from build123d import *

# Parameters (mm, degrees)
EXTRUDE1_DEPTH = 6


with BuildPart() as part:
    # Sketch1 → Extrude1 (new body)
    with BuildSketch(Plane(origin=(0, 0, 0), x_dir=(1, 0, 0), z_dir=(0, 1, 0))):
        Polygon((1.154700538, 2), (-1.154700538, 2), (-2.309401077, 0), (-1.154700538, -2), (1.154700538, -2), (2.309401077, 0), align=None)
    extrude(amount=EXTRUDE1_DEPTH)

    # Sketch3 → Cut-Revolve1 (revolve, cut)
    with BuildSketch(Plane(origin=(0, 0, 0), x_dir=(0, 0, -1), z_dir=(1, 0, 0)), mode=Mode.PRIVATE) as cut_revolve1_sk:
        Polygon((1.5, 6), (1, 5.5), (1, 0.5), (1.5, 0), (0, 0), (0, 6), align=None)
    revolve(cut_revolve1_sk.sketch.rotate(Axis((0, 6, 0), (0, -1, 0)), 180), axis=Axis((0, 6, 0), (0, -1, 0)), mode=Mode.SUBTRACT)

    # Sketch4 → Cut-Revolve3 (revolve, cut)
    with BuildSketch(Plane(origin=(0, 0, 0), x_dir=(0, 0, -1), z_dir=(1, 0, 0))):
        Polygon((2, 6), (4.5, 6), (4.5, 3.5), align=None)
        Polygon((2, 0), (4.5, 0), (4.5, 2.5), align=None)
    revolve(axis=Axis((0, 0, 0), (0, 1, 0)), mode=Mode.SUBTRACT)


solid = part.part
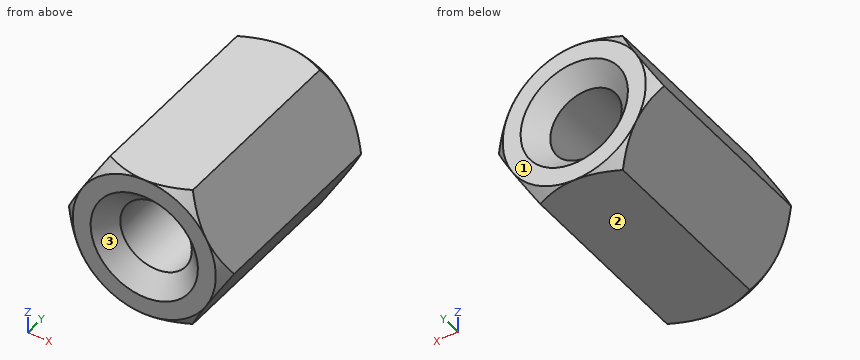
Part model, mm, in its own coordinate system. Face numbers are marked on the shaded views. Give positions to 0.01 mm unless a question says otherwise; leave off trailing zeros. Loops run counter-clockwise (first coordinate to the right, second up) from the corner with the lowest first, then second, coordinate; pieces in that order, holes last. Notation, with made-up numbers: M 46,28.25 L 53,28.25 A35 ccw 53,63.25 Z; hole C -24,-15.5 d10. An arc over 180 degrees is marked long. Put each result on its own line as item: value. Start each with the question number.
1) Probe probe 1 along X at (y, z) = (1, -0.75); probe 2 along X at (y, z) = (3, -0.85); probe 3 along Z at (x, y) = (0.45, 0.75). List the from-to ranges inside material, lowest first.
2) Saw through at A-A (y = 1). List the corners of the cut face in (x, z), then the cut area to 3 significant figures.
3) Pull direction Z, two halves, no side cores. Call the marked faces 1, 2 and 3: +Z half, -Z half, draft (parallel to the pull), parting line (faces both ways), or undercut.
Numbers:
1. probe 1: -1.88 to -0.66, 0.66 to 1.88
1. probe 2: -1.82 to -0.53, 0.53 to 1.82
1. probe 3: -2 to -0.89, 0.89 to 2
2. outline: M -2.31,0 L -1.15,-2 L 1.15,-2 L 2.31,0 L 1.15,2 L -1.15,2 Z; hole C 0,0 d2
2. area: 10.7 mm^2
3. face 1: draft
3. face 2: -Z half
3. face 3: undercut
